Could you check a few things on this model? Use its own coordinates, in mm. Coordinates: 2 decimals unless noted, no trailing zeros. Write each loop counter-clockwise with the first axis right and the second up, starting at its lowest first coordinate (ties: lowest second). Pieces come first, ordered by that corner, then holes.
Item 1: I want a section at C-C on z = 168.25. Please give me the cut outline in (x, y), then the cut area to 3 significant figures.
Item 2: For P1, Ø7.5, axis at x = 25.4, y = 0, coming from the -Z side, with a flat end and sliding along its axis, tell me the tip position at first contact or that it passes through.
Item 3: Thinking about a two-plate mould opening in Y: for faces 1 (the flat face through (-1, 25.4, 165)), 2 (the flat face through (50.8, 0, 165)), 3 (the flat face through (-1, -25.4, 165)), 4 (the cylindrical face through (19.056, 0.279, 164.922)), which applies, +Y half, -Y half, draft (parallel to the pull), parting line (faces both ways), or undercut?
Item 4: I want a section at B-B on x = 25.4. Please give me the cut outline in (y, z), then the cut area to 3 significant figures.
Item 5: I want a section at A-A on y = 0. Please give me the cut outline in (x, z).
Item 6: If I drill on probe 1 along Y at (x, z) = (25.4, 165); probe 2 along X at (y, z) = (-3, 163); probe 3 along Y at (x, z) = (31, 176), over which ranges is the centre line in solid material (lowest first)?
from build123d import *

# Parameters (mm, degrees)
F1_W     = 101.6
F1_H     = 50.8
F1_R     = 6.35
F2_DEPTH = 25.4


with BuildPart() as f2:
    # F1 (on offset) → F2 (new body)
    with BuildSketch(Plane.XY.offset(152.4)):
        Rectangle(F1_W, F1_H)
        with Locations((25.4, 0)):
            Circle(F1_R, mode=Mode.SUBTRACT)
    extrude(amount=F2_DEPTH)


solid = f2.part
Response values:
1. outline: (-50.8, -25.4) - (50.8, -25.4) - (50.8, 25.4) - (-50.8, 25.4) - close; hole circle Ø12.7 at (25.4, 0)
1. area: 5,030 mm2
2. P1: passes through
3. face 1: +Y half
3. face 2: draft
3. face 3: -Y half
3. face 4: undercut
4. outline: (-25.4, 152.4) - (-6.35, 152.4) - (-6.35, 177.8) - (-25.4, 177.8) - close; (6.35, 152.4) - (25.4, 152.4) - (25.4, 177.8) - (6.35, 177.8) - close
4. area: 968 mm2
5. outline: (-50.8, 152.4) - (19.05, 152.4) - (19.05, 177.8) - (-50.8, 177.8) - close; (31.75, 152.4) - (50.8, 152.4) - (50.8, 177.8) - (31.75, 177.8) - close
6. probe 1: y = -25.4 to -6.35, 6.35 to 25.4
6. probe 2: x = -50.8 to 19.8, 31 to 50.8
6. probe 3: y = -25.4 to -2.99, 2.99 to 25.4
